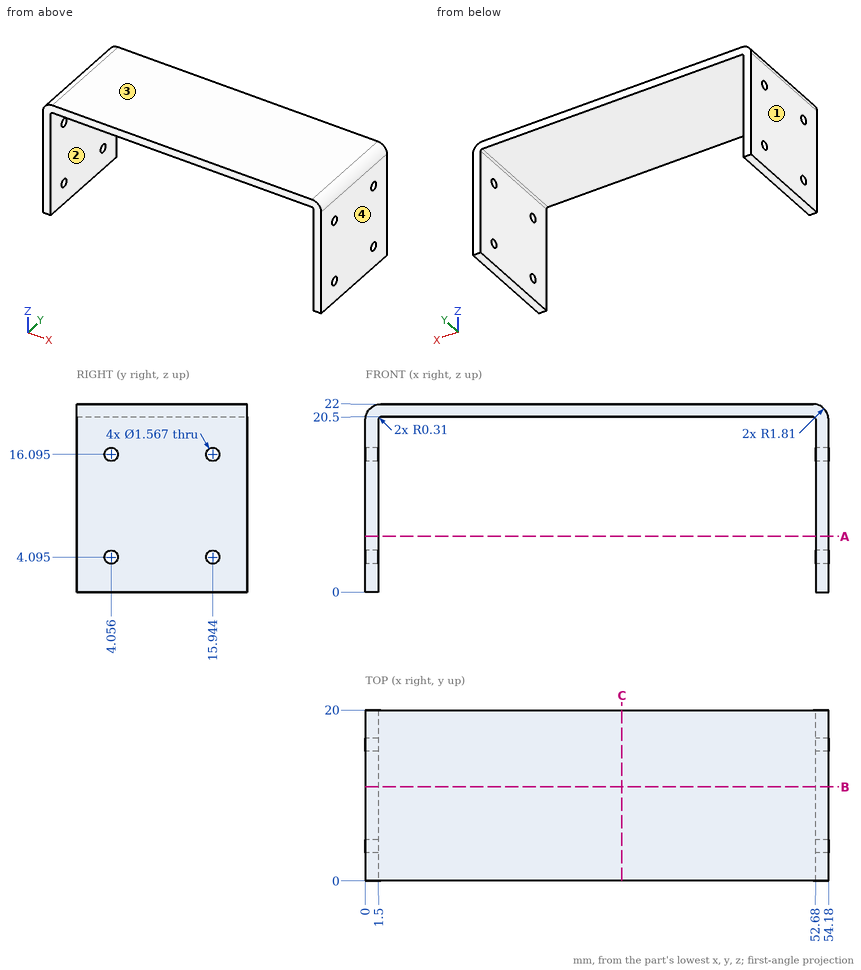
Part print with two shaded views. Sizes in mm from the minimum x, y, z corner. Round coordinates to 2 decimals unless told otherwise and drop trailing zeros. Write each loop counter-clockwise with the first axis right and the second up, starting at its lowest first coordinate (ties: lowest second). Pieces come first, ordered by that corner, then holes. Notation, with made-up numbers: (-23.5, 15) -> (-7.5, 15) arc R27 ccw to (-7.5, 47) -> close; hole circle Ø3 at (66.25, -12). An arc over 180 degrees is marked (long way). Put each result on its own line as item: value.
Item 1: Slice it at A-A, the plane z = 6.5. Give the cut face in (x, y).
Here are the results:
outline: (0, 0) -> (1.5, 0) -> (1.5, 20) -> (0, 20) -> close; (52.68, 0) -> (54.18, 0) -> (54.18, 20) -> (52.68, 20) -> close
Item 2: Flat gauge pin, fed straight in: P1, Ø6, axis at x = 18, y = 7.5, coming from the -Z side. Where does the tip first touch, or does it go through?
Here are the results:
P1: stops at z = 20.5
Item 3: Slice it at B-B, the plane y = 11. Give the cut face in (x, z).
Here are the results:
outline: (0, 0) -> (1.5, 0) -> (1.5, 20.19) arc R0.31 cw to (1.81, 20.5) -> (52.37, 20.5) arc R0.31 cw to (52.68, 20.19) -> (52.68, 0) -> (54.18, 0) -> (54.18, 20.19) arc R1.81 ccw to (52.37, 22) -> (1.81, 22) arc R1.81 ccw to (0, 20.19) -> close
Item 4: Two-plate mould, pull along X, no slides. Class the marked faces 1, 2, 3 and 4: pulls with the +X half, pulls with the -X half, needs draft (parallel to the pull), parting line crosses it, or undercut.
Here are the results:
face 1: pulls with the -X half
face 2: undercut
face 3: needs draft
face 4: pulls with the +X half
Item 5: Slice it at C-C, the plane x = 30. Give the cut face in (y, z).
Here are the results:
outline: (0, 20.5) -> (20, 20.5) -> (20, 22) -> (0, 22) -> close
Item 6: Wall check: probe 1 along X at (y, z) = (18.5, 11.5); probe 2 along Z at (x, y) = (18.5, 8.25). Give the ranges that are in metal, low to high. Write a range as from..to.
Here are the results:
probe 1: x = 0..1.5, 52.68..54.18
probe 2: z = 20.5..22
